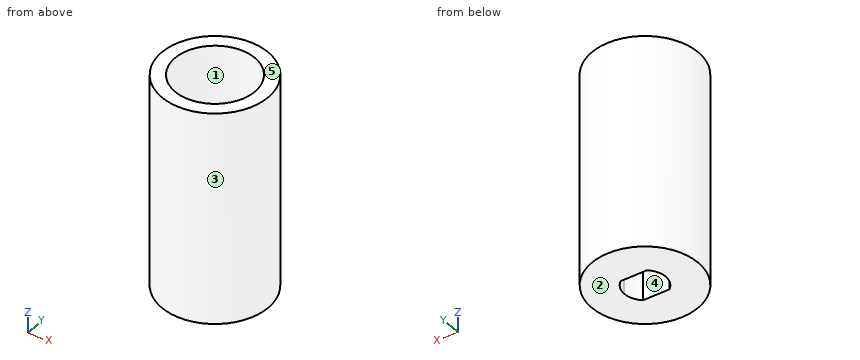
```python
from build123d import *

# Parameters (mm, degrees)
F0_R     = 4
F1_DEPTH = 16
F3_D     = 6
F3_DEPTH = 8
F3_TIP   = 1.8025818571


with BuildPart() as f1:
    # F0 (on Top) → F1 (new body)
    with BuildSketch(Plane.XY):
        Circle(F0_R)
        with BuildLine():
            ThreePointArc((-1.55, 0), (-1.4005641377, 0.6640181445), (-0.9810708435, 1.2))
            Line((-0.9810708435, 1.2), (0.9810708435, 1.2))
            ThreePointArc((0.9810708435, 1.2), (1.4005641377, 0.6640181445), (1.55, 0))
            ThreePointArc((1.55, 0), (1.4005641377, -0.6640181445), (0.9810708435, -1.2))
            Line((0.9810708435, -1.2), (-0.9810708435, -1.2))
            ThreePointArc((-0.9810708435, -1.2), (-1.4005641377, -0.6640181445), (-1.55, 0))
        make_face(mode=Mode.SUBTRACT)
    extrude(amount=F1_DEPTH)

    # F3
    with Locations(Plane.XY.offset(16)):
        with Locations((0, 0)):
            Hole(F3_D / 2, depth=F3_DEPTH)
            with Locations((0, 0, -(F3_DEPTH + F3_TIP / 2))):  # 118° drill point
                Cone(0, F3_D / 2, F3_TIP, mode=Mode.SUBTRACT)


solid = f1.part
```
The model under review builds one solid part; all positions refer to its coordinate system, in mm. Face numbers are marked on the shaded views. A direction names the side the tool comes from. Give positions to 0.01 mm unless a question says otherwise; leave off trailing zeros. Write each loop counter-clockwise with the first axis right and the second up, starting at its lowest first coordinate (ties: lowest second). Pieces come first, ordered by that corner, then holes. Notation, with made-up numbers: M -9,24.25 L 37,24.25 A19 cw 37,31.25 Z; hole C 57.25,88.25 d3. An arc over 180 degrees is marked long. Write each question's results on one line, items separated by ' | '. Start each with the question number.
1. Insertion check: pin 1 Ø1.5 at (x, z) = (-2, 2) entering from -Y. The pin has a flat end and moves straight along its axis. Give the tip position at first contact, or say it passes through.
2. We need section D-D (x = 3.5). Write out the cut boundary in (y, z), and give its area (3 significant figures).
3. For probe 1 along Y at (x, z) = (0, 11); probe 2 along X at (y, z) = (2, 10.25); probe 3 along X at (y, z) = (1.5, 2), list the stretches that pass through material, from the lowest coordinate up. Write a range as [from, to].
4. Mouldability with a two-part tool opening along Y and no side actions: class the marked faces 1, 2 and 3 as released by +Y, released by -Y, zero draft, split by the parting line, or undercut.
5. We need section C-C (z = 14.75). Write out the cut boundary in (x, y).
6. For the marked faces 4 and 5, list the 3-axis set-ups (+Z, -Z, +X, -X, +Y, -Y) from which the entire face can be reached by the end or side of a thin tool; tool diameter is ignored.
7. We need section A-A (x = 0). Write out the cut boundary in (y, z), and give its area (3 significant figures).
8. We need section B-B (z = 1.5). Write out the cut boundary in (x, y), and give its area (3 significant figures).
Results found:
1) pin 1: stops at y = -3.8
2) outline: M -1.94,0 L 1.94,0 L 1.94,16 L -1.94,16 Z | area: 62.0 mm^2
3) probe 1: y = [-4, -3], [3, 4] | probe 2: x = [-3.46, -2.24], [2.24, 3.46] | probe 3: x = [-3.71, 3.71]
4) face 1: undercut | face 2: zero draft | face 3: split by the parting line
5) outline: C 0,0 d8; hole C 0,0 d6
6) face 4: +Z, -Z | face 5: +Z, +X, -X, +Y, -Y
7) outline: M -4,0 L -1.2,0 L -1.2,6.92 L -3,8 L -3,16 L -4,16 Z; M 1.2,0 L 4,0 L 4,16 L 3,16 L 3,8 L 1.2,6.92 Z | area: 58.9 mm^2
8) outline: C 0,0 d8; hole M -0.98,-1.2 L 0.98,-1.2 A1.55 ccw 0.98,1.2 L -0.98,1.2 A1.55 ccw Z | area: 43.7 mm^2
